```python
from build123d import *

# Parameters (mm, degrees)
SKETCH_1_R      = 27.5
EXTRUDE_1_DEPTH = 30
SKETCH_2_R      = 25
EXTRUDE_2_DEPTH = 22
SKETCH_3_R      = 27.5
EXTRUDE_3_DEPTH = 13


with BuildPart() as part:
    # Эскиз1 → Бобышка-Вытянуть1 (new body)
    with BuildSketch(Plane(origin=(0, 0, 0), x_dir=(1, 0, 0), z_dir=(0, 1, 0))):
        with Locations(Location((0, 0, 0), (0, 0, 270))):
            Circle(SKETCH_1_R)
    extrude(amount=EXTRUDE_1_DEPTH)

    # Эскиз2 → Бобышка-Вытянуть2 (add)
    with BuildSketch(Plane(origin=(0, 30, 0), x_dir=(1, 0, 0), z_dir=(0, 1, 0))):
        with Locations(Location((0, 0, 0), (0, 0, 270))):
            Circle(SKETCH_2_R)
    extrude(amount=EXTRUDE_2_DEPTH)

    # Эскиз3 → Бобышка-Вытянуть3 (add)
    with BuildSketch(Plane(origin=(0, 52, 0), x_dir=(1, 0, 0), z_dir=(0, 1, 0))):
        with Locations(Location((0, 0, 0), (0, 0, 270))):
            Circle(SKETCH_3_R)
    extrude(amount=EXTRUDE_3_DEPTH)


solid = part.part
```
Build history of the part. All positions in model axes, mm. A direction names the side the tool comes from. Give positions to 0.01 mm unless a question says otherwise; leave off trailing zeros. Loops run counter-clockwise (first coordinate to the right, second up) from the corner with the lowest first, then second, coordinate; pieces in that order, holes last.
1) Drop flat-ended pins along their axis: P1, Ø1, axis at y = 14, z = 16.5, coming from the -X side; P2, Ø10, axis at y = 27, z = -18.5, coming from the -X side; P3, Ø8, axis at y = 54.5, z = 16.5, coming from the -X side. Give the stop position or say it passes through.
Values follow:
P1: stops at x = -22.37
P2: stops at x = -23.96
P3: stops at x = -24.49
2) Band-saw the part on B-B on x = 0. List the corners of the cut face in (y, z), then the cut area to 4 significant figures.
Values follow:
outline: (0, -27.5) - (30, -27.5) - (30, -25) - (52, -25) - (52, -27.5) - (65, -27.5) - (65, 27.5) - (52, 27.5) - (52, 25) - (30, 25) - (30, 27.5) - (0, 27.5) - close
area: 3,465 mm2
3) Two-plate mould, pull along Y, no slides. Class faces 3 (the face through (-24.397, 14.79, 12.69)), 4 (the face through (-22.3, 30, 12.1)), 5 (the face through (0, 65, 0)): released by +Y, released by -Y, zero draft, split by the parting line, or undercut.
Values follow:
face 3: zero draft
face 4: undercut
face 5: released by +Y
4) Band-saw the part on C-C on y = 27. List the corners of the cut face in (x, z), then the cut area to 3 significant figures.
Values follow:
outline: circle Ø55 at (0, 0)
area: 2,380 mm2
5) Probe line 1 along Y through (x, z) = (22.5, -13); line 2 along X through (y, z) = (16, 1); line 3 along Z through (x, y) = (-0.5, 5). List the from-to ranges inside material, lowest first.
Values follow:
line 1: y = 0 to 30, 52 to 65
line 2: x = -27.48 to 27.48
line 3: z = -27.5 to 27.5
6) 3-axis set-ups, long thin cutter, end or side, ignore diameter. For faces 1 (the face through (-22.3, 52, 12.1)), 2 (the face through (0, 0, 0)): which of +Z, -Z, +X, -X, +Y, -Y reach the whole face in a straight line?
Values follow:
face 1: none
face 2: +Z, -Z, +X, -X, -Y
7) Band-saw the part on A-A on z = 0. List the corners of the cut face in (x, y).
Values follow:
outline: (-27.5, 0) - (27.5, 0) - (27.5, 30) - (25, 30) - (25, 52) - (27.5, 52) - (27.5, 65) - (-27.5, 65) - (-27.5, 52) - (-25, 52) - (-25, 30) - (-27.5, 30) - close
